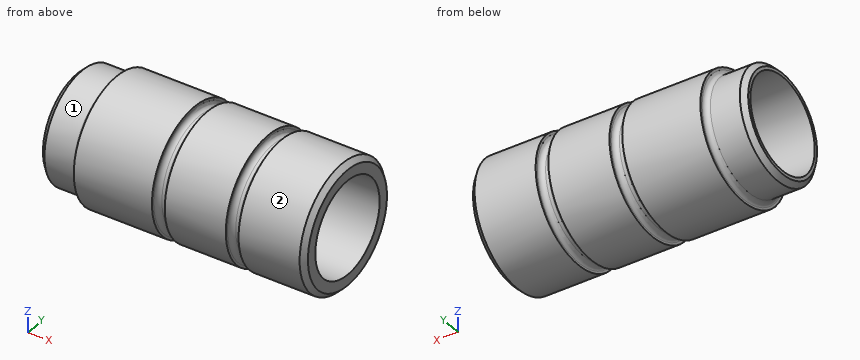
```python
from build123d import *


with BuildPart() as part:
    # Sketch1 → Revolve1 (revolve)
    with BuildSketch(Plane.XY):
        with BuildLine():
            Line((0, 9.525), (-55, 9.525))
            Line((-55, 9.525), (-55, 10.2))
            Line((-55, 10.2), (-54, 11.2))
            Line((-54, 11.2), (-48, 11.2))
            ThreePointArc((-48, 11.2), (-47.292893219, 11.492893219), (-47, 12.2))
            Line((-47, 12.2), (-47, 12.7))
            Line((-47, 12.7), (-31.08207122, 12.7))
            Line((-31.08207122, 12.7), (-31.08207122, 12.2))
            ThreePointArc((-31.08207122, 12.2), (-30.789178001, 11.492893219), (-30.08207122, 11.2))
            Line((-30.08207122, 11.2), (-29.477097815, 11.2))
            ThreePointArc((-29.477097815, 11.2), (-28.769991033, 11.492893219), (-28.477097815, 12.2))
            Line((-28.477097815, 12.2), (-28.477097815, 12.7))
            Line((-28.477097815, 12.7), (-16.04103561, 12.7))
            Line((-16.04103561, 12.7), (-16.04103561, 12.2))
            ThreePointArc((-16.04103561, 12.2), (-15.748142391, 11.492893219), (-15.04103561, 11.2))
            Line((-15.04103561, 11.2), (-14.436062205, 11.2))
            ThreePointArc((-14.436062205, 11.2), (-13.728955423, 11.492893219), (-13.436062205, 12.2))
            Line((-13.436062205, 12.2), (-13.436062205, 12.7))
            Line((-13.436062205, 12.7), (-1, 12.7))
            Line((-1, 12.7), (0, 11.7))
            Line((0, 11.7), (0, 9.525))
        make_face()
    revolve(axis=Axis((19.168296655, 0, 0), (-1, 0, 0)))


solid = part.part
```
The listing builds one solid part. Answer for the finished solid, in the listing's coordinates (mm). Face numbers are marked on the shaded views. A direction names the side the tool comes from. Give positions to 0.01 mm unless a question says otherwise; leave off trailing zeros. Order: outer loops, then holes, each group sorted by start corner. A loop starts at its lowest first (then second) coordinate and runs counter-clockwise, first axis right, second up.
Item 1: Which of the six approach directions +Z, -Z, +X, -X, +Y, -Y give full straight-line access (tool end or side, diameter ignored) to the marked faces 1 and 2?
From the geometry:
face 1: -X
face 2: +X, -X
Item 2: Given pin 1 Ø4 at (x, z) = (-38.5, -4) entering from +Y; pin 2 Ø8 at (x, y) = (-26.5, 9) entering from +Z; pin 3 Ø4 at (x, z) = (-15.5, 7) entering from -Y, each flat-ended and moving along its own axis, determine where each tip first touches the part or whether it passes through.
From the geometry:
pin 1: stops at y = 12.54
pin 2: stops at z = 11.67
pin 3: stops at y = -11.64
Item 3: The part is cut by section A-A, the plane x = -37. Give the vertices of the cut face in (y, z) (3 decimals).
From the geometry:
outline: circle Ø25.4 at (0, 0); hole circle Ø19.05 at (0, 0)
Item 4: Find the intervals of material crossed by probe 1 along Z at (x, y) = (-41, 0) (3 decimals); probe 2 along X at (y, z) = (5.75, -10), in increasing order.
From the geometry:
probe 1: z = -12.7 to -9.525, 9.525 to 12.7
probe 2: x = -47.25 to -30.83, -28.73 to -15.79, -13.69 to 0
